Source: CAD feature listing. Evaluate the final solid. Frame: model axes, mm. A direction names the side the tool comes from. Give positions to 0.01 mm unless a question says otherwise; leave off trailing zeros. Order: outer loops, then holes, each group sorted by start corner. A loop starts at its lowest first (then second) coordinate and runs counter-clockwise, first axis right, second up. Notation, with made-up numbers: M 69,33 L 104,33 A19 cw 104,64 Z; hole C 25.5,55 d2. An arc over 180 degrees is marked long. One line per question, with ' | ' between items. Start each with the question number.
Autodesk Inventor part; units mm, degrees
ref_plane "YZ Plane" through (0, 0, 0) normal (1, 0, 0) x (0, 1, 0)
ref_plane "XZ Plane" through (0, 0, 0) normal (0, 1, 0) x (-1, 0, 0)
ref_plane "XY Plane" through (0, 0, 0) normal (0, 0, 1) x (1, 0, 0)
sketch "Sketch1" plane through (0, 0, 0) normal (0, 0, 1) x (1, 0, 0)
  line L0 (15, -15) -> (-15, -15)
  line L1 (-15, -15) -> (-15, 15)
  line L2 (-15, 15) -> (15, 15)
  line L3 (15, 15) -> (15, -15)
  line L4 (15, -15) -> (-15, 15) construction
  line L5 (-15, -15) -> (15, 15) construction
  point P0 (0, 0)
  dimension "d0" = 30
  dimension "d1" = 30
extrude "Extrusion1" add sketch "Sketch1" against normal blind 20
sketch "Sketch2" plane through (-15, 15, 0) normal (0, 1, 0) x (1, 0, 0)
  line L0 (30, 0) -> (30, 20)
  line L1 (0, 5) -> (30, 5)
  line L2 (30, 5) -> (30, 10)
  line L3 (30, 10) -> (0, 10)
  line L4 (0, 10) -> (0, 5)
  line L5 (0, 5) -> (30, 10) construction
  line L6 (30, 5) -> (0, 10) construction
  line L7 (0, 20) -> (30, 20)
  point P0 (15, 0)
  point P1 (15, 7.5)
  dimension "d4" = 5
  dimension "d13" = 10
extrude "Extrusion2" cut sketch "Sketch2" against normal blind 11
sketch "Sketch3" plane through (-15, -15, 0) normal (0, -1, 0) x (1, 0, 0)
  line L0 (30, 0) -> (30, -20)
  line L1 (0, -5) -> (30, -5)
  line L2 (30, -5) -> (30, -10)
  line L3 (30, -10) -> (0, -10)
  line L4 (0, -10) -> (0, -5)
  line L5 (0, -5) -> (30, -10) construction
  line L6 (30, -5) -> (0, -10) construction
  line L7 (30, -20) -> (0, -20)
  point P0 (15, 0)
  point P1 (15, -7.5)
  dimension "d7" = 5
  dimension "d14" = 10
extrude "Extrusion3" cut sketch "Sketch3" against normal blind 11
sketch "Sketch4" plane through (0, 0, 0) normal (0, 0, 1) x (1, 0, 0)
  circle A0 centre (0, 0) radius 4
  dimension "d10" = 8
extrude "Extrusion4" cut sketch "Sketch4" against normal blind 5
sketch "Sketch6" plane through (0, 0, 0) normal (0, 0, 1) x (1, 0, 0)
  line L0 (15, 15) -> (-15, 15)
  line L1 (-15, 15) -> (-15, -15)
  circle A0 centre (0, 0) radius 4
  line L2 (15, 15) -> (-15, 15)
  line L3 (-15, 15) -> (-15, -15)
  line L4 (-15, -15) -> (15, -15)
  line L5 (15, -15) -> (15, 15)
extrude "Extrusion5" add sketch "Sketch6" along normal blind 10
sketch "Sketch7" plane through (15, -15, -20) normal (1, 0, 0) x (0, 0, -1)
  line L0 (-10, 30) -> (-10, 19)
  line L1 (-10, 19) -> (-15, 19)
  line L2 (-30, 19) -> (-15, 19)
  point P0 (-12.5, 15)
sketch "Sketch8" plane through (15, -15, -20) normal (1, 0, 0) x (0, 0, -1)
  line L0 (-15, 0) -> (-30, 0)
  line L1 (-22.5, 0) -> (-22.5, 10) construction
  line L2 (-21.1875, 0) -> (-21.1875, 10)
  line L3 (-23.8125, 10) -> (-23.8125, 0)
  arc A0 (-23.8125, 0) -> (-21.1875, 0) centre (-22.5, 0) ccw
  arc A1 (-21.1875, 10) -> (-23.8125, 10) centre (-22.5, 10) ccw
  point P0 (-20, 15)
  point P1 (-22.5, 5)
  dimension "d17" = 10
  dimension "d18" = 2.625
extrude "Extrusion6" cut sketch "Sketch8" against normal through all contours L0 L3 A1 L2
sketch "Sketch9" plane through (0, 0, 10) normal (0, 0, 1) x (1, 0, 0)
  line L0 (15, -15) -> (15, -5)
  line L1 (15, -15) -> (5, -15)
  line L2 (-15, -15) -> (15, -15)
  line L3 (5, -15) -> (5, -10)
  circle A0 centre (5, -10) radius 2
  line L4 (0, 0) -> (0, -15)
  line L5 (-15, -15) -> (-5, -15)
  line L6 (15, -15) -> (-15, -15)
  line L7 (-5, -15) -> (-5, -10)
  circle A1 centre (-5, -10) radius 2
  dimension "d21" = 10
  dimension "d22" = 5
  dimension "d23" = 4
extrude "Extrusion7" cut sketch "Sketch9" against normal blind 15
fillet "Fillet1" radius 2 17 edges at (0, 15, 10) (15, 0, 10) (-15, 0, 10) (-15, 15, 2.5) (0, 15, -5) (15, 15, 2.5) (15, -15, -1.9062) (15, -15, 6.9062) (15, 0, -20) (15, 15, -15) (0, 15, -20) (-15, 15, -15) (0, 15, -10) (15, -15, -15) (-15, 0, -20) (-15, -15, -15) (-15, -15, 6.9062)
properties part number "Corredera" material "Iron, Cast"
Item 1: Line query: line 1 (X direction, y = -10, z = 6.25); line 2 (Z direction, x = 7, y = 9); line 3 (X direction, y = 0, z = 5). Output: solid intervals per line, ascending.
Item 2: Reachability of faces 4 (the flat face through (0, -10, 1.188)), 5 (the flat face through (0, 9, -5)), 6 (the cylindrical face through (-5, -8, 7)) from +Z, -Z, +X, -X, +Y, -Y: full face, straight path, thin tool, end or side. Return the list, or none.
Item 3: Cut plane C-C on y = 7.25. Return the cut outline in (x, z).
Item 4: Mould query, pull axis Z, two halves, no side actions, for faces 1 (the cylindrical face through (-14.4, -0.8, -19.43)), 2 (the flat face through (0, 15, -15)), 3 (the flat face through (0, -10, 3.812)). Classes: pulls with the +Z half, pulls with the -Z half, needs draft (parallel to the pull), parting line crosses it, or undercut.
Item 5: Cut plane B-B on x = -5. Return the cut outline in (y, z) (1 decimal).
Item 6: Pin query (flat end, axial travel): pin 1 Ø8 at (x, y) = (6, -10) entering from +Z; pin 2 Ø2.5 at (x, z) = (2, -8) entering from -Y; pin 3 Ø3 at (x, y) = (-5, -10) entering from +Z; pin 4 Ø1.5 at (x, z) = (-6.5, -7.5) entering from +Y. Return the tip coordinate at first contact, or that it passes through.
Item 7: Cut plane D-D on y = -10. Count the separate pieces of the cut face and the enclosed holes in it, and give its area (3 significant figures).
Item 8: Cut plane A-A on z = 6. Return the cut outline in (x, y), and give its area (3 significant figures).
Results are:
1) line 1: x = -15 to -7, -3 to 3, 7 to 15 | line 2: z = -20 to -10, -5 to 10 | line 3: x = -15 to -4, 4 to 15
2) face 4: +X, -X, -Y | face 5: +X, -X, +Y | face 6: +Z
3) outline: M -15,-18 A2 ccw -13,-20 L 13,-20 A2 ccw 15,-18 L 15,-10 L -15,-10 Z; M -15,-5 L 15,-5 L 15,8 A2 ccw 13,10 L -13,10 A2 ccw -15,8 Z
4) face 1: pulls with the -Z half | face 2: needs draft | face 3: undercut
5) outline: M -15,-20 L 13,-20 A2 ccw 15,-18 L 15,-12 A2 ccw 13,-10 L 4,-10 L 4,-5 L 13,-5 A2 ccw 15,-3 L 15,8 A2 ccw 13,10 L -8,10 L -8,3.8 L -5,3.8 A1.3 cw -5,1.2 L -8,1.2 L -8,-5 L -4,-5 L -4,-10 L -15,-10 Z; M -15,-5 L -12,-5 L -12,1.2 L -15,1.2 Z; M -15,3.8 L -12,3.8 L -12,10 L -15,10 Z
6) pin 1: stops at z = 10 | pin 2: stops at y = -4 | pin 3: stops at z = -10 | pin 4: stops at y = 4
7) separate pieces: 7 | enclosed holes: 0 | area: 569 mm2
8) outline: M -15,-13 A2 ccw -13,-15 L 13,-15 A2 ccw 15,-13 L 15,13 A2 ccw 13,15 L -13,15 A2 ccw -15,13 Z; hole C -5,-10 d4; hole C 0,0 d8; hole C 5,-10 d4 | area: 821 mm2
